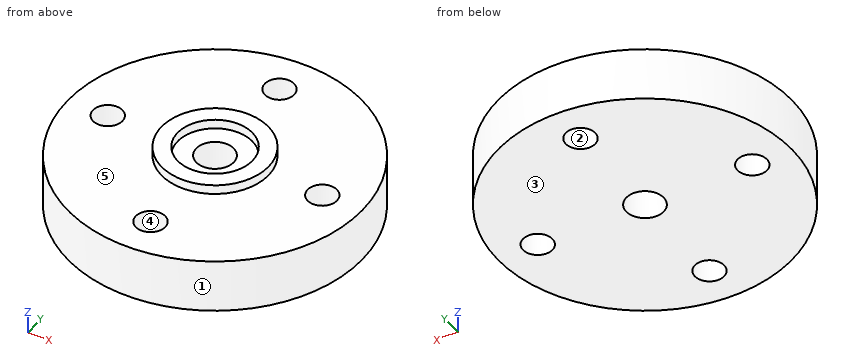
from build123d import *

# Parameters (mm, degrees)
ESQUISSE1_R      = 11
ESQUISSE1_R_2    = 1.1
EXTRUSION1_DEPTH = 4
ESQUISSE2_R      = 4
ESQUISSE2_R_2    = 2.8
EXTRUSION3_DEPTH = 0.7
EXTRUSION4_REACH = 6
ESQUISSE3_R      = 1.4


with BuildPart() as part:
    # Esquisse1 → Extrusion1 (new body)
    with BuildSketch(Plane.XY):
        Circle(ESQUISSE1_R)
        with Locations((0, 8)):
            Circle(ESQUISSE1_R_2, mode=Mode.SUBTRACT)
        with Locations((-8, 0)):
            Circle(ESQUISSE1_R_2, mode=Mode.SUBTRACT)
        with Locations((8, 0)):
            Circle(ESQUISSE1_R_2, mode=Mode.SUBTRACT)
        with Locations((0, -8)):
            Circle(ESQUISSE1_R_2, mode=Mode.SUBTRACT)
    extrude(amount=EXTRUSION1_DEPTH)

    # Esquisse2 → Extrusion3 (add)
    with BuildSketch(Plane.XY.offset(4)):
        Circle(ESQUISSE2_R)
        Circle(ESQUISSE2_R_2, mode=Mode.SUBTRACT)
    extrude(amount=EXTRUSION3_DEPTH)

    # Esquisse3 → Extrusion4 (cut, up to next)
    with BuildSketch(Plane.XY.offset(4), mode=Mode.PRIVATE) as extrusion4_sk1:
        Circle(ESQUISSE3_R)
    extrusion4_tool1 = extrude(extrusion4_sk1.sketch, amount=-EXTRUSION4_REACH, mode=Mode.PRIVATE) & part.part
    add(extrusion4_tool1.solids().sort_by_distance((0, 0, 4))[0], mode=Mode.SUBTRACT)


solid = part.part
Source: CAD feature listing. Evaluate the final solid. Frame: model axes, mm. Face numbers are marked on the shaded views. A direction names the side the tool comes from. Give positions to 0.01 mm unless a question says otherwise; leave off trailing zeros. Write each loop counter-clockwise with the first axis right and the second up, starting at its lowest first coordinate (ties: lowest second). Pieces come first, ordered by that corner, then holes. Notation, with made-up numbers: M 84,13 L 112,13 A28 ccw 112,45 Z; hole C -8,-18 d9. An arc over 180 degrees is marked long. Return JSON: item names as keys, results as strings. Group by question number.
1) Pull-direction query (Y, two-part tool) for the marked faces 1, 2 and 3; classes: pulls with the +Y half, pulls with the -Y half, needs draft (parallel to the pull), parting line crosses it, or undercut.
2) Material intervals for line 1 along Y through (x, z) = (0, 2.7); line 2 along Y through (x, z) = (-0.75, 2.7); line 3 along Z through (x, y) = (-6.25, 7), sorted ascending. Write a range as [from, to].
3) Cut plane C-C, the plane z = 4.4. Output: boundary loops of the cut face in (x, y), plus the area to 3 significant figures.
4) Pin query (flat end, axial travel): P1, Ø2, axis at x = 8, y = 7.5, coming from the +Z side; P2, Ø1.5, axis at x = -2.5, z = 2.5, coming from the +Y side. Return the tip coordinate at first contact, or that it passes through.
5) Cut plane A-A, the plane x = 0. Output: boundary loops of the cut face in (y, z).
6) Cut plane D-D, the plane x = -8. Output: boundary loops of the cut face in (y, z).
7) Set-up query: the marked faces 4 and 5. Return all of +Z, -Z, +X, -X, +Y, -Y with unobstructed straight access to the full face (end or side cutting, diameter ignored); none if empty.
Recorded:
{
 "1": {"face 1": "parting line crosses it", "face 2": "undercut", "face 3": "needs draft"},
 "2": {"line 1": "y = [-11, -9.1], [-6.9, -1.4], [1.4, 6.9], [9.1, 11]", "line 2": "y = [-10.97, -8.8], [-7.2, -1.18], [1.18, 7.2], [8.8, 10.97]", "line 3": "z = [0, 4]"},
 "3": {"outline": "C 0,0 d8; hole C 0,0 d5.6", "area": "25.6 mm²"},
 "4": {"P1": "stops at z = 4", "P2": "stops at y = 10.86"},
 "5": {"outline": "M -11,0 L -9.1,0 L -9.1,4 L -11,4 Z; M -6.9,0 L -1.4,0 L -1.4,4 L -2.8,4 L -2.8,4.7 L -4,4.7 L -4,4 L -6.9,4 Z; M 1.4,0 L 6.9,0 L 6.9,4 L 4,4 L 4,4.7 L 2.8,4.7 L 2.8,4 L 1.4,4 Z; M 9.1,0 L 11,0 L 11,4 L 9.1,4 Z"},
 "6": {"outline": "M -7.55,0 L -1.1,0 L -1.1,4 L -7.55,4 Z; M 1.1,0 L 7.55,0 L 7.55,4 L 1.1,4 Z"},
 "7": {"face 4": "+Z, -Z", "face 5": "+Z"}
}
